```python
from build123d import *

# Parameters (mm, degrees)
SKETCH1_R           = 2.24506403
SKETCH1_R_2         = 2.5
BOSS_EXTRUDE1_DEPTH = 10


with BuildPart() as part:
    # Sketch1 → Boss-Extrude1 (new body)
    with BuildSketch(Plane(origin=(0, 0, 0), x_dir=(1, 0, 0), z_dir=(0, 1, 0))):
        with BuildLine():
            ThreePointArc((10, -100), (0, -110), (-10, -100))
            Line((-10, -100), (-10, 100))
            ThreePointArc((-10, 100), (0, 110), (10, 100))
            Line((10, 100), (10, -100))
        make_face()
        with Locations(Location((0, 100, 0), (0, 0, 270))):
            Circle(SKETCH1_R, mode=Mode.SUBTRACT)
        with Locations(Location((0, -100, 0), (0, 0, 270))):
            Circle(SKETCH1_R_2, mode=Mode.SUBTRACT)
    extrude(amount=BOSS_EXTRUDE1_DEPTH)


solid = part.part
```
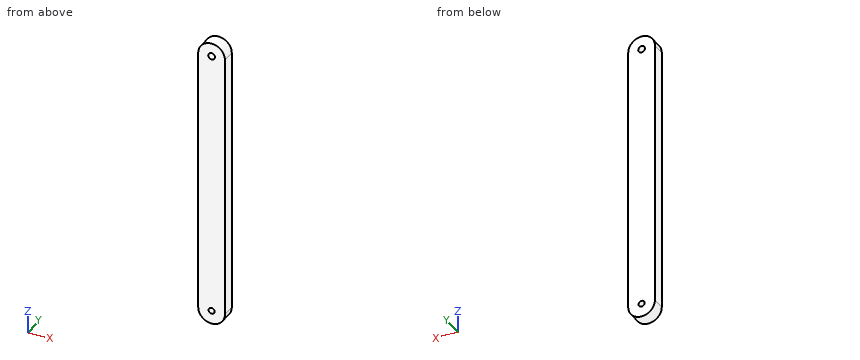
Part model, mm, in its own coordinate system. Coordinates: 2 decimals unless noted, no trailing zeros. Order: outer loops, then holes, each group sorted by start corner. A loop starts at its lowest first (then second) coordinate and runs counter-clockwise, first axis right, second up. Notation, with made-up numbers: (87.25, 79.5) - (96.25, 79.5) arc R12 cw to (96.25, 89.5) - close; hole circle Ø2 at (19, 29). An arc over 180 degrees is marked (long way). Return JSON: item names as keys, results as strings. Group by question number.
Item 1: Pin check, flat tips, straight feed: pin 1 (3 mm diameter, centred on x = 0, z = 100, fed in from -Y); pin 2 (2 mm diameter, centred on x = 1.5, y = 5, fed in from +Z). Stop position of each tip, or through.
Item 2: Drill centre lines: probe 1 along X at (y, z) = (5.25, -100); probe 2 along X at (y, z) = (7, 100); probe 3 along Z at (x, y) = (-8.5, 8.75). Where is each one in solid material? Low to high. Write a range as from..to.
Item 3: Cut at A-A (x = 0). List the corners of the cut face in (y, z), plus the area to 3 significant figures.
Item 4: Cut at B-B (y = 7.75). List the corners of the cut face in (x, z).
Check values:
{
 "1": {"pin 1": "passes through", "pin 2": "stops at z = 109.99"},
 "2": {"probe 1": "x = -10..-2.25, 2.25..10", "probe 2": "x = -10..-2.5, 2.5..10", "probe 3": "z = -105.27..105.27"},
 "3": {"outline": "(0, -110) - (10, -110) - (10, -102.25) - (0, -102.25) - close; (0, -97.75) - (10, -97.75) - (10, 97.5) - (0, 97.5) - close; (0, 102.5) - (10, 102.5) - (10, 110) - (0, 110) - close", "area": "2,110 mm2"},
 "4": {"outline": "(-10, -100) arc R10 ccw to (10, -100) - (10, 100) arc R10 ccw to (-10, 100) - close; hole circle Ø5 at (0, 100); hole circle Ø4.49 at (0, -100)"}
}
